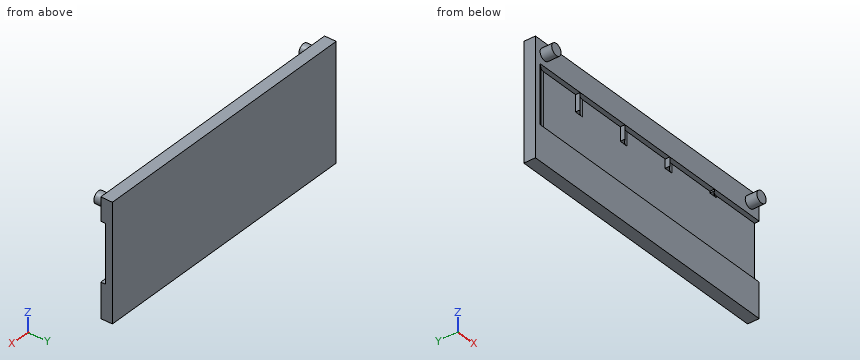
```python
from build123d import *

# Parameters (mm, degrees)
SKETCH1_W               = 120
SKETCH1_H               = 50
BOSS_EXTRUDE1_DEPTH     = 5
CUT_EXTRUDE1_DEPTH      = 131.096118313
CUT_EXTRUDE1_DEPTH_BACK = 120
SKETCH2_W               = 25
SKETCH2_H               = 2
BOSS_EXTRUDE2_DEPTH     = 0.75
BOSS_EXTRUDE3_DEPTH     = 3.8
BOSS_EXTRUDE4_DEPTH     = 5.95
BOSS_EXTRUDE6_DEPTH     = 7.1
SKETCH10_R              = 2.5
BOSS_EXTRUDE7_DEPTH     = 5
BOSS_EXTRUDE8_DEPTH     = 25
SKETCH12_W              = 2.455775423
SKETCH12_H              = 2
BOSS_EXTRUDE9_DEPTH     = 25
FILLET1_R               = 4


with BuildPart() as part:
    # Sketch1 → Boss-Extrude1 (new body)
    with BuildSketch(Plane(origin=(0, 0, 0), x_dir=(1, 0, 0), z_dir=(0, 1, 0))):
        with Locations((8.146341463, 25)):
            Rectangle(SKETCH1_W, SKETCH1_H)
    extrude(amount=BOSS_EXTRUDE1_DEPTH)

    # Sketch2 → Cut-Extrude1 (cut, two sides: drawn at the far end of the back side and taken through both)
    with BuildSketch(Plane(origin=(68.146341463, 0, 0), x_dir=(0, 0, -1), z_dir=(1, 0, 0)).offset(-CUT_EXTRUDE1_DEPTH_BACK)):
        with Locations((22.5, 1)):
            Rectangle(SKETCH2_W, SKETCH2_H)
    extrude(amount=CUT_EXTRUDE1_DEPTH + CUT_EXTRUDE1_DEPTH_BACK, mode=Mode.SUBTRACT)

    # Sketch5 → Boss-Extrude2 (add)
    with BuildSketch(Plane(origin=(0, 0, -10), x_dir=(-1, 0, 0), z_dir=(0, 0, -1))):
        Polygon((-44.148415926, 0), (-46.148415926, 2), (-44.148415926, 2), align=None)
    extrude(amount=BOSS_EXTRUDE2_DEPTH)

    # Sketch6 → Boss-Extrude3 (add)
    with BuildSketch(Plane(origin=(0, 0, -10), x_dir=(-1, 0, 0), z_dir=(0, 0, -1))):
        Polygon((-20.178332659, 0), (-20.178332659, 2), (-22.178332659, 2), align=None)
    extrude(amount=BOSS_EXTRUDE3_DEPTH)

    # Sketch7 → Boss-Extrude4 (add)
    with BuildSketch(Plane(origin=(0, 0, -10), x_dir=(-1, 0, 0), z_dir=(0, 0, -1))):
        Polygon((3.853324248, 0), (3.853324248, 2), (1.853324248, 2), align=None)
    extrude(amount=BOSS_EXTRUDE4_DEPTH)

    # Sketch9 → Boss-Extrude6 (add)
    with BuildSketch(Plane(origin=(0, 0, -10), x_dir=(-1, 0, 0), z_dir=(0, 0, -1))):
        Polygon((27.849622994, 0), (27.853491393, 2), (25.853491393, 2), align=None)
    extrude(amount=BOSS_EXTRUDE6_DEPTH)

    # Sketch10 → Boss-Extrude7 (add)
    with BuildSketch(Plane.XZ):
        with Locations(Location((-46.853658537, -5, 0), (0, 0, 270))):
            Circle(SKETCH10_R)
        with Locations(Location((63.146341463, -5, 0), (0, 0, 270))):
            Circle(SKETCH10_R)
    extrude(amount=BOSS_EXTRUDE7_DEPTH)

    # Sketch11 → Boss-Extrude8 (add)
    with BuildSketch(Plane(origin=(0, 0, -10), x_dir=(-1, 0, 0), z_dir=(0, 0, -1))):
        Polygon((49.397883114, 0), (49.397883114, 2), (46.169924942, 2), align=None)
    extrude(amount=BOSS_EXTRUDE8_DEPTH)

    # Sketch12 → Boss-Extrude9 (add)
    with BuildSketch(Plane(origin=(0, 0, -10), x_dir=(-1, 0, 0), z_dir=(0, 0, -1))):
        with Locations((50.625770825, 1)):
            Rectangle(SKETCH12_W, SKETCH12_H)
    extrude(amount=BOSS_EXTRUDE9_DEPTH)

    # Fillet1
    fillet1_edges = [part.edges().sort_by_distance(p)[0] for p in [
        (-46.169924942, 2, -22.5),
        (46.148415926, 2, -10.375),
        (22.178332659, 2, -11.9),
        (-1.853324248, 2, -12.975),
        (-25.853491393, 2, -13.55),
    ]]
    fillet(fillet1_edges, radius=FILLET1_R)


solid = part.part
```
Geometry check sheet. Reference: the model listing, model coordinates, mm. Round coordinates to 2 decimals unless told otherwise and drop trailing zeros. Order: outer loops, then holes, each group sorted by start corner. A loop starts at its lowest first (then second) coordinate and runs counter-clockwise, first axis right, second up. Notation, with made-up numbers: (-16.5, 83) - (42.5, 83) arc R29 ccw to (42.5, 120) - close; hole circle Ø8 at (75.25, 76.25). An arc over 180 degrees is marked (long way). Use a Markdown table: item, result. Add a question column.
1) Section check D-D (z = -43). Record the cut outline in (x, y).
2) Section check B-B (x = 13.5). Record the cut outline in (y, z).
3) Thickness scan on line 1 along X through (y, z) = (0.5, -11); line 2 along Z through (x, y) = (-20.5, 1.75); line 3 along Y through (x, z) = (25, -25.5). Record the ranges inside material, lowest first.
4) Section check A-A (z = -22). Record the cut outline in (x, y).
5) Gauge pin test, flat ends, axial feed: P1, Ø2, axis at x = 35.5, z = -29.5, coming from the -Y side; P2, Ø15, axis at x = 18.5, z = -36.5, coming from the -Y side. Record the tip position at first contact, or that the pin passes through.
6) Section check C-C (z = -5). Record the cut outline in (x, y).
Established:
| question | item | result |
|---|---|---|
| 1 | outline | (-51.85, 0) - (68.15, 0) - (68.15, 5) - (-51.85, 5) - close |
| 2 | outline | (0, -50) - (5, -50) - (5, 0) - (0, 0) - (0, -10) - (2, -10) - (2, -35) - (0, -35) - close |
| 3 | line 1 | -51.85 to -48.59, -27.85 to -27.35, -3.85 to -3.35, 20.18 to 20.68 |
| 3 | line 2 | -50 to -35, -10 to 0 |
| 3 | line 3 | 2 to 5 |
| 4 | outline | (-51.85, 0) - (-49.4, 0) - (-47.14, 1.4) arc R4 cw to (-45.03, 2) - (68.15, 2) - (68.15, 5) - (-51.85, 5) - close |
| 5 | P1 | y = 2 |
| 5 | P2 | y = 0 |
| 6 | outline | (-51.85, 0) - (-49.35, 0) - (-49.35, -5) - (-44.35, -5) - (-44.35, 0) - (60.65, 0) - (60.65, -5) - (65.65, -5) - (65.65, 0) - (68.15, 0) - (68.15, 5) - (-51.85, 5) - close |
